Can you work these out from the model? Positions are in its coordinate system, mm. Give positions to 0.01 mm unless a question says otherwise; leave off trailing zeros. Write each loop counter-clockwise with the first axis right and the second up, starting at its lowest first coordinate (ties: lowest second). Pieces come first, ordered by that corner, then holes. Notation, with made-up numbers: M 54.5,40.25 L 66.5,40.25 A14 ccw 66.5,61.25 Z; hole C 33,48.25 d5. An arc over 180 degrees is marked long. Answer as CSV lines item,"result". Start each with the question number.
```python
from build123d import *

# Parameters (mm, degrees)
BOSS_EXTRUDE1_DEPTH = 6
FILLET1_R           = 1


with BuildPart() as part:
    # Sketch1 → Boss-Extrude1 (new body)
    with BuildSketch(Plane(origin=(0, 0, 0), x_dir=(1, 0, 0), z_dir=(0, 1, 0))):
        Polygon((0, 0), (6.5, 11.258330249), (13, 0), align=None)
    extrude(amount=BOSS_EXTRUDE1_DEPTH)

    # Fillet1
    fillet1_edges = [part.edges().sort_by_distance(p)[0] for p in [
        (3.25, 6, -5.629165125),
        (3.25, 0, -5.629165125),
        (6.5, 6, 0),
        (9.75, 0, -5.629165125),
        (6.5, 0, 0),
        (0, 3, 0),
        (6.5, 3, -11.258330249),
        (13, 3, 0),
        (9.75, 6, -5.629165125),
    ]]
    fillet(fillet1_edges, radius=FILLET1_R)


solid = part.part
```
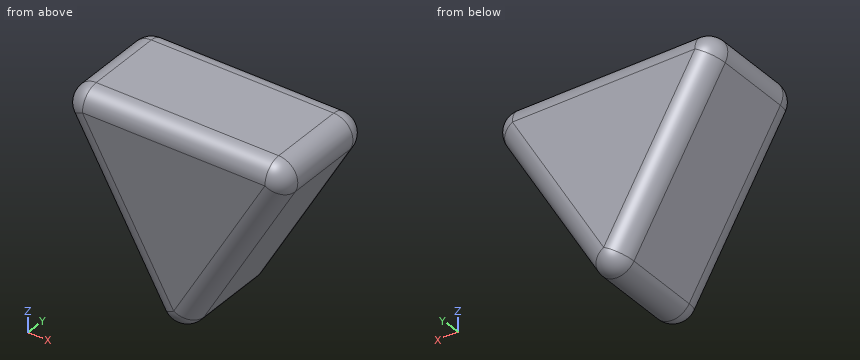
1) I want a section at A-A, the plane y = 3.75. Please give me the cut outline in (x, z).
2) I need wall thicknesses on L1, parallel to X at y = 4.25, z = -3.5; L2, parallel to X at y = 0.5, z = -2; L3, parallel to Z at x = 9.5, y = 2.5. Which ranges of each line are inside material? Lowest first, please. Write a range as from..to.
3) I'm going to push a flat-ended pin straight in: P1, Ø2, axis at x = 5, y = 3, coming from the -Z side. Where does the tip first touch, or does it pass through?
4) I want a section at B-B, the plane y = 5.5. Please give me the cut outline in (x, z), then the cut area to 3 significant figures.
Values found:
1,outline,"M 0.87,-1.5 L 5.63,-9.76 A1 ccw 7.37,-9.76 L 12.13,-1.5 A1 ccw 11.27,0 L 1.73,0 A1 ccw Z"
2,L1,"x = 2.02..10.98"
2,L2,"x = 1.31..11.69"
2,L3,"z = -6.06..0"
3,P1,"stops at z = -10.12"
4,outline,"M 0.98,-1.43 L 5.75,-9.69 A0.87 ccw 7.25,-9.69 L 12.02,-1.43 A0.87 ccw 11.27,-0.13 L 1.73,-0.13 A0.87 ccw Z"
4,area,"66.5 mm²"
